Design review of the part shown in the three views and the two pictorial views. Dimensions are in mm from the part's minimum x, y and z. Coordinates: 2 decimals unless noted, no trailing zeros. Write each loop counter-clockwise with the first axis right and the second up, starting at its lowest first coordinate (ties: lowest second). Pieces come first, ordered by that corner, then holes. Notation, with made-up numbers: M 72.5,-13.75 L 97.5,-13.75 A15 cw 97.5,8.25 Z; hole C -30,-1 d5. An arc over 180 degrees is marked long. Answer as a JSON object with one key per item and string values.
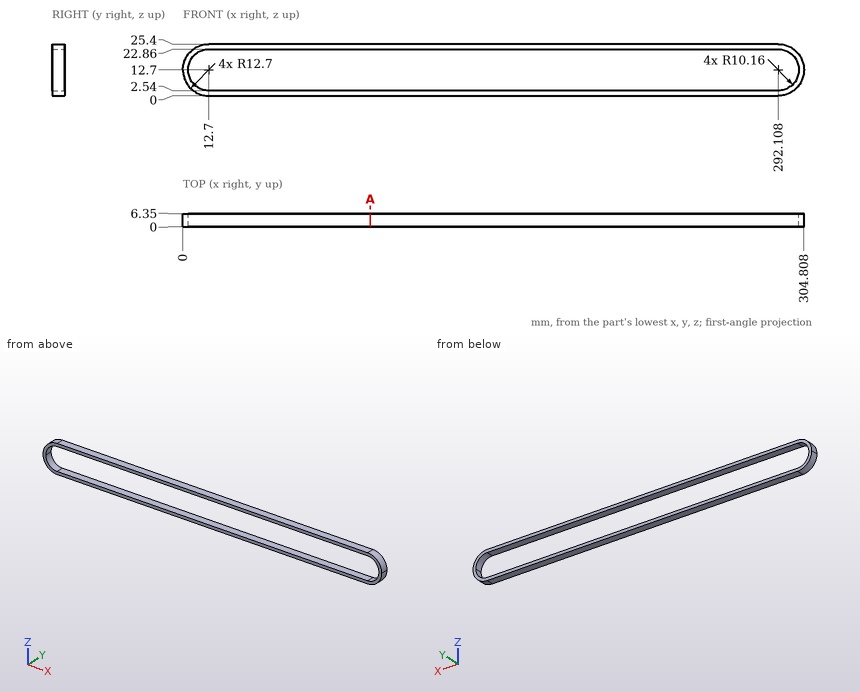
(1) Add section A-A on x = 92. Give the boundary of the cut face in (y, z).
Results list:
{"outline": "M 0,0 L 6.35,0 L 6.35,2.54 L 0,2.54 Z; M 0,22.86 L 6.35,22.86 L 6.35,25.4 L 0,25.4 Z"}
(2) Wall thickness on line 1 along Z through (x, y) = (277.5, 2.75); line 2 along X through (y, z) = (2.75, 13.75) (1 decimal); line 3 along X through (y, z) = (5, 12.75): over which ranges is each line inside the solid? List them lowest first. Write a range as from..to.
Results list:
{"line 1": "0..2.54, 22.86..25.4", "line 2": "0..2.6, 302.2..304.8", "line 3": "0..2.54, 302.27..304.81"}
(3) For pin 1 Ø2 at (y, z) = (4.5, 19) entering from -X; pin 2 Ø10 at (x, z) = (108.5, 11.5) entering from +Y, all flat-tipped, find the tip position at first contact; note any pin that passes through.
Results list:
{"pin 1": "x = 1.16", "pin 2": "through"}
